```python
from build123d import *

# Parameters (mm, degrees)
F0_W           = 7.14375
F0_H           = 25.4
F3_D           = 12.7
F3_DEPTH       = 12.7
F3_CSINK_D     = 14.2875
F3_CSINK_ANGLE = 90
F3_TIP         = 3.8154649308
F5_DEPTH       = 12.7
F6_SIZE        = 0.254


with BuildPart() as f1:
    # F0 (on Front) → F1 (revolve)
    with BuildSketch(Plane.XZ):
        with Locations((-3.571875, -12.7)):
            Rectangle(F0_W, F0_H)
    revolve(axis=Axis((0, 0, -12.7), (0, 0, -1)))

    # F3
    with Locations(Plane.XY):
        with Locations((0, 0)):
            CounterSinkHole(F3_D / 2, F3_CSINK_D / 2, depth=F3_DEPTH, counter_sink_angle=F3_CSINK_ANGLE)
            with Locations((0, 0, -(F3_DEPTH + F3_TIP / 2))):  # 118° drill point
                Cone(0, F3_D / 2, F3_TIP, mode=Mode.SUBTRACT)

    # F4 (on face) → F5 (cut)
    with BuildSketch(Plane(origin=(0, 0, -25.4), x_dir=(1, 0, 0), z_dir=(0, 0, -1))):
        Polygon((-3.175, -1.3151280605), (-3.175, -3.175), (-1.3151280605, -3.175), align=None)
        Polygon((1.3151280605, -3.175), (-1.3151280605, -3.175), (0, -4.4901280605), align=None)
        Polygon((3.175, -1.3151280605), (1.3151280605, -3.175), (3.175, -3.175), align=None)
        Polygon((-3.175, 3.175), (-3.175, 1.3151280605), (-1.3151280605, 3.175), align=None)
        Polygon((0, 4.4901280605), (-1.3151280605, 3.175), (1.3151280605, 3.175), align=None)
        Polygon((1.3151280605, 3.175), (3.175, 1.3151280605), (3.175, 3.175), align=None)
        Polygon((-4.4901280605, 0), (-3.175, -1.3151280605), (-3.175, 1.3151280605), align=None)
        Polygon((-3.175, -1.3151280605), (-1.3151280605, -3.175), (1.3151280605, -3.175), (3.175, -1.3151280605), (3.175, 1.3151280605), (1.3151280605, 3.175), (-1.3151280605, 3.175), (-3.175, 1.3151280605), align=None)
        Polygon((3.175, 1.3151280605), (3.175, -1.3151280605), (4.4901280605, 0), align=None)
    extrude(amount=-F5_DEPTH, mode=Mode.SUBTRACT)

    # F6
    f6_edges = [f1.edges().sort_by_distance(p)[0] for p in [
        (7.14375, 0, -25.4),
    ]]
    chamfer(f6_edges, length=F6_SIZE)


solid = f1.part
```
Can you work these out from the model? Positions are in its coordinate system, mm. A direction names the side the tool comes from. Give positions to 0.01 mm unless a question says otherwise; leave off trailing zeros. Loops run counter-clockwise (first coordinate to the right, second up) from the corner with the lowest first, then second, coordinate; pieces in that order, holes last. Notation, with made-up numbers: M 46,64 L 83,64 A11 cw 83,76 Z; hole C -3.5,-26 d7. An arc over 180 degrees is marked long. Use CSV: the item, a comma, the result in double quotes. Start each with the question number.
1. If we mould it in two halves opening along X, with no side actions, what happens to faces 1 (the face through (-3.175, 2, -20)), 2 (the face through (-1, -4, -25.4))? For each: released by +X, released by -X, zero draft, split by the parting line, or undercut.
2. Imagine slicing it at B-B, the plane z = -7.75. Write out the boundary of the cut face in (x, y).
3. If I drill on L1, parallel to Y at x = 0, z = -5.5; L2, parallel to X at y = 2.5, z = -15 (3 decimals); L3, parallel to X at y = 1.75, z = -7, over which ranges is the centre line in solid material (lowest first)?
4. On a 3-axis mill with a long thin cutter (end or side, diameter ignored), from which of +Z, -Z, +X, -X, +Y, -Y can I reach the whole of each face in a straight line? I mean faces 3 (the face through (-0.67, 3.82, -19.69)), 4 (the face through (1.38, -6.2, -6.83)). Say none if no direction works.
5. Imagine slicing it at A-A, the plane z = -15.75. Write out the boundary of the cut face in (x, y) (1 decimal).
6. For P1, Ø1.5, axis at y = -2.5, z = -16, coming from the -X side; P2, Ø2, axis at y = 2, z = -20, coming from the +X side; P3, Ø2, axis at y = 2, z = -17.5, coming from the -X side, each with a flat end and sliding along its axis, tell me the tip position at first contact or that it passes through.
Response values:
1,face 1,"undercut"
1,face 2,"zero draft"
2,outline,"C 0,0 d14.29; hole C 0,0 d12.7"
3,L1,"-7.14 to -6.35, 6.35 to 7.14"
3,L2,"-6.692 to -3.175, 3.175 to 6.692"
3,L3,"-6.93 to -6.1, 6.1 to 6.93"
4,face 3,"+Z, -Z"
4,face 4,"+Z"
5,outline,"C 0,0 d14.3; hole M -4.5,0 L -3.2,-1.3 L -3.2,-3.2 L -1.3,-3.2 L 0,-4.5 L 1.3,-3.2 L 3.2,-3.2 L 3.2,-1.3 L 4.5,0 L 3.2,1.3 L 3.2,3.2 L 1.3,3.2 L 0,4.5 L -1.3,3.2 L -3.2,3.2 L -3.2,1.3 Z"
6,P1,"x = -6.93"
6,P2,"x = 7.07"
6,P3,"x = -7.07"
